Input: part model. Units: mm. Frame: model coordinates. A direction names the side the tool comes from. Round coordinates to 2 decimals unless told otherwise and drop trailing zeros. Loops run counter-clockwise (first coordinate to the right, second up) from the corner with the lowest first, then second, coordinate; pieces in that order, holes last. Notation, with made-up numbers: (54, 84) - (108, 84) arc R32 ccw to (108, 120) - close; hole circle Ø5 at (12.25, 44.5). An arc over 180 degrees is marked (long way). One line per question, with ' | ' between items. Start each with the question number.
from build123d import *

# Parameters (mm, degrees)
SKETCH079_R          = 9.5
PAD028_DEPTH         = 8
POCKET026_DEPTH      = 70.546983
POCKET026_DEPTH_BACK = 70.546983
POLARPATTERN_COUNT   = 8
SKETCH081_W          = 10
SKETCH081_H          = 4
PAD030_DEPTH         = 8
SKETCH082_R          = 1.8
POCKET_DEPTH         = 11.501


with BuildPart() as part:
    # Sketch079 → Pad028 (new body, symmetric)
    with BuildSketch(Plane.XZ):
        Circle(SKETCH079_R)
    extrude(amount=PAD028_DEPTH, both=True)

    # Sketch078 → Pocket026 (cut, two sides)
    with BuildSketch(Plane.XZ) as pocket026_sk:
        with BuildLine():
            Line((0.866025, -7.5), (6.928203, 3))
            ThreePointArc((6.928203, 3), (6.928203, 4), (6.062178, 4.5))
            Line((6.062178, 4.5), (-6.062178, 4.5))
            ThreePointArc((-6.062178, 4.5), (-6.928203, 4), (-6.928203, 3))
            Line((-6.928203, 3), (-0.866025, -7.5))
            ThreePointArc((-0.866025, -7.5), (0, -8), (0.866025, -7.5))
        make_face()
    pocket026 = extrude(amount=-POCKET026_DEPTH, mode=Mode.SUBTRACT) + extrude(pocket026_sk.sketch, amount=POCKET026_DEPTH_BACK, mode=Mode.SUBTRACT)

    # PolarPattern: Pocket026 ×8 about axis
    polarpattern_axis = Axis((0, 0, 0), (0, 1, 0))
    for i in range(1, POLARPATTERN_COUNT):
        add(pocket026.rotate(polarpattern_axis, i * 360 / POLARPATTERN_COUNT), mode=Mode.SUBTRACT)

    # Sketch081 → Pad030 (join, symmetric)
    with BuildSketch(Plane.XZ):
        with Locations((14, 0)):
            Rectangle(SKETCH081_W, SKETCH081_H)
    extrude(amount=PAD030_DEPTH, both=True)

    # Sketch082 (on Face6 of Pad030) → Pocket (cut, through all)
    with BuildSketch(Plane(origin=(0, 0, 2), x_dir=(-1, 0, 0), z_dir=(0, 0, 1))):
        with Locations((-16.5, 5)):
            Circle(SKETCH082_R)
        with Locations((-16.5, -5)):
            Circle(SKETCH082_R)
    extrude(amount=-POCKET_DEPTH, mode=Mode.SUBTRACT)


with BuildPart() as part_1:
    # Body011 placement: moved
    add(part.part.moved(Location((-12, 0, 2))))


solid = part_1.part
(1) Pull-direction query (Z, two-part tool) for faces 3 (the face through (-4.27, -0.11, 4.06)), 4 (the face through (2, 0, 4)), 5 (the face through (-4.276, -0.112, -0.085)), 6 (the face through (7, 0, 2)); classes: released by +Z, released by -Z, zero draft, split by the parting line, or undercut.
(2) Reachability of faces 1 (the face through (-4, 8, 1)), 2 (the face through (-8.013, -0.112, -4.935)) from +Z, -Z, +X, -X, +Y, -Y: full face, straight path, thin tool, end or side. Return the list, or none.
(3) Section A-A, the plane z = 2. Output: boundary loops of the cut face in (x, y).
(4) Section D-D, the plane y = 5. Give the number of separate pieces and of enclosed holes in the cut face, plus the area to 3 significant figures.
(5) Line query: line 1 along Y through (x, z) = (4.5, 0.8); line 2 along X through (y, z) = (-5, 1.3); line 3 along X through (y, z) = (5, 2.3). Output: solid intervals per line, ascending. Write a range as from..to.
(6) Section B-B, the plane x = -12. Output: boundary loops of the cut face in (y, z).
(7) Pin query (flat end, axial travel): P1, Ø10, axis at x = -18, z = -1, coming from the -Y side; P2, Ø4, axis at x = -7, y = -6, coming from the -Z side; P3, Ø6, axis at x = 4.5, y = -5, coming from the +Z side; P4, Ø3, axis at x = 1.5, y = -4, coming from the -Z side. Return the tip coordinate at first contact, or that it passes through.
(8) Section C-C, the plane x = 4.5. Output: boundary loops of the cut face in (y, z), plus the area to 3 significant figures.
Derived:
1) face 3: undercut | face 4: released by +Z | face 5: undercut | face 6: zero draft
2) face 1: +Z, -Z, +X, -X, +Y | face 2: +Y, -Y
3) outline: (-21.5, -8) - (-20, -8) - (-20, 8) - (-21.5, 8) - close; (-4, -8) - (7, -8) - (7, 8) - (-4, 8) - close; hole circle Ø3.6 at (4.5, -5); hole circle Ø3.6 at (4.5, 5)
4) separate pieces: 2 | enclosed holes: 1 | area: 115 mm²
5) line 1: y = -8..-6.8, -3.2..3.2, 6.8..8 | line 2: x = -21.47..-19.71, -4.29..2.7, 6.3..7 | line 3: x = -21.5..-19.95, -4.05..2.7, 6.3..7
6) outline: (-8, -7.5) - (8, -7.5) - (8, -6) - (-8, -6) - close; (-8, 10) - (8, 10) - (8, 11.5) - (-8, 11.5) - close
7) P1: stops at y = -8 | P2: stops at z = -7.01 | P3: stops at z = 4 | P4: stops at z = 0
8) outline: (-8, 0) - (-6.8, 0) - (-6.8, 4) - (-8, 4) - close; (-3.2, 0) - (3.2, 0) - (3.2, 4) - (-3.2, 4) - close; (6.8, 0) - (8, 0) - (8, 4) - (6.8, 4) - close | area: 35.2 mm²
